from build123d import *

# Parameters (mm, degrees)
SKETCH1_W                      = 765
SKETCH1_H                      = 550
BASE_FLANGE1_DEPTH             = 1.8
EDGE_FLANGE1_STRIP_W           = 8.6732
EDGE_FLANGE1_STRIP_H           = 1.8
EDGE_FLANGE1_STRIP_CUT_DEPTH   = 550
EDGE_FLANGE1_STRIP_2_W         = 8.6732
EDGE_FLANGE1_STRIP_2_H         = 1.8
EDGE_FLANGE1_STRIP_CUT_2_DEPTH = 550
EDGE_FLANGE1_DEPTH             = 550
EDGE_FLANGE1_BEND_DEPTH        = 550
EDGE_FLANGE2_STRIP_W           = 8.6732
EDGE_FLANGE2_STRIP_H           = 1.8
EDGE_FLANGE2_STRIP_CUT_DEPTH   = 550
EDGE_FLANGE2_STRIP_2_W         = 8.6732
EDGE_FLANGE2_STRIP_2_H         = 1.8
EDGE_FLANGE2_STRIP_CUT_2_DEPTH = 550
EDGE_FLANGE2_DEPTH             = 550
EDGE_FLANGE2_BEND_DEPTH        = 550
SKETCH18_R                     = 3.5
CUT_EXTRUDE1_DEPTH             = 10


# Sheet-metal steps are written as plain solids
with BuildPart() as part:
    # Sketch1 → Base-Flange1 (new body)
    with BuildSketch(Plane(origin=(0, 0, 0), x_dir=(0, 0, -1), z_dir=(1, 0, 0))):
        Rectangle(SKETCH1_W, SKETCH1_H)
    extrude(amount=-BASE_FLANGE1_DEPTH)

    # Edge-Flange1 strip (across the edge) → Edge-Flange1 strip cut (cut)
    with BuildSketch(Plane(origin=(0, 275, 382.5), x_dir=(0, 0, -1), z_dir=(0, -1, 0))):
        with Locations((-1.8, -0.9)):
            Rectangle(EDGE_FLANGE1_STRIP_W, EDGE_FLANGE1_STRIP_H)
    extrude(amount=EDGE_FLANGE1_STRIP_CUT_DEPTH, mode=Mode.SUBTRACT)

    # Edge-Flange1 strip 2 (across the edge) → Edge-Flange1 strip cut 2 (cut)
    with BuildSketch(Plane(origin=(0, -275, -382.5), x_dir=(0, 0, 1), z_dir=(0, 1, 0))):
        with Locations((-1.8, -0.9)):
            Rectangle(EDGE_FLANGE1_STRIP_2_W, EDGE_FLANGE1_STRIP_2_H)
    extrude(amount=EDGE_FLANGE1_STRIP_CUT_2_DEPTH, mode=Mode.SUBTRACT)

    # Edge-Flange1 section (across the edge) → Edge-Flange1 (add)
    with BuildSketch(Plane(origin=(0, 275, 382.5), x_dir=(0, 0, -1), z_dir=(0, -1, 0))):
        with BuildLine():
            Line((0, 0.7366), (0, 48.2))
            Line((0, 48.2), (1.8, 48.2))
            Line((1.8, 48.2), (1.8, 0.7366))
            ThreePointArc((1.8, 0.7366), (2.015745145, 0.215745145), (2.5366, 0))
            Line((2.5366, 0), (2.5366, -1.8))
            ThreePointArc((2.5366, -1.8), (0.742952939, -1.057047061), (0, 0.7366))
        make_face()
    extrude(amount=EDGE_FLANGE1_DEPTH)

    # Edge-Flange1 section 2 (across the edge) → Edge-Flange1 bend (add)
    with BuildSketch(Plane(origin=(0, -275, -382.5), x_dir=(0, 0, 1), z_dir=(0, 1, 0))):
        with BuildLine():
            Line((0, 0.7366), (0, 48.2))
            Line((0, 48.2), (1.8, 48.2))
            Line((1.8, 48.2), (1.8, 0.7366))
            ThreePointArc((1.8, 0.7366), (2.015745145, 0.215745145), (2.5366, 0))
            Line((2.5366, 0), (2.5366, -1.8))
            ThreePointArc((2.5366, -1.8), (0.742952939, -1.057047061), (0, 0.7366))
        make_face()
    extrude(amount=EDGE_FLANGE1_BEND_DEPTH)

    # Edge-Flange2 strip (across the edge) → Edge-Flange2 strip cut (cut)
    with BuildSketch(Plane(origin=(48.2, 275, -382.5), x_dir=(-1, 0, 0), z_dir=(0, -1, 0))):
        with Locations((-3.6, -0.9)):
            Rectangle(EDGE_FLANGE2_STRIP_W, EDGE_FLANGE2_STRIP_H)
    extrude(amount=EDGE_FLANGE2_STRIP_CUT_DEPTH, mode=Mode.SUBTRACT)

    # Edge-Flange2 strip 2 (across the edge) → Edge-Flange2 strip cut 2 (cut)
    with BuildSketch(Plane(origin=(48.2, -275, 382.5), x_dir=(-1, 0, 0), z_dir=(0, 1, 0))):
        with Locations((-3.6, -0.9)):
            Rectangle(EDGE_FLANGE2_STRIP_2_W, EDGE_FLANGE2_STRIP_2_H)
    extrude(amount=EDGE_FLANGE2_STRIP_CUT_2_DEPTH, mode=Mode.SUBTRACT)

    # Edge-Flange2 section (across the edge) → Edge-Flange2 (add)
    with BuildSketch(Plane(origin=(48.2, 275, -382.5), x_dir=(-1, 0, 0), z_dir=(0, -1, 0))):
        with BuildLine():
            Line((-1.8, 0.7366), (-1.8, 28.2))
            Line((-1.8, 28.2), (0, 28.2))
            Line((0, 28.2), (0, 0.7366))
            ThreePointArc((0, 0.7366), (0.215745145, 0.215745145), (0.7366, 0))
            Line((0.7366, 0), (0.7366, -1.8))
            ThreePointArc((0.7366, -1.8), (-1.057047061, -1.057047061), (-1.8, 0.7366))
        make_face()
    extrude(amount=EDGE_FLANGE2_DEPTH)

    # Edge-Flange2 section 2 (across the edge) → Edge-Flange2 bend (add)
    with BuildSketch(Plane(origin=(48.2, -275, 382.5), x_dir=(-1, 0, 0), z_dir=(0, 1, 0))):
        with BuildLine():
            Line((-1.8, 0.7366), (-1.8, 28.2))
            Line((-1.8, 28.2), (0, 28.2))
            Line((0, 28.2), (0, 0.7366))
            ThreePointArc((0, 0.7366), (0.215745145, 0.215745145), (0.7366, 0))
            Line((0.7366, 0), (0.7366, -1.8))
            ThreePointArc((0.7366, -1.8), (-1.057047061, -1.057047061), (-1.8, 0.7366))
        make_face()
    extrude(amount=EDGE_FLANGE2_BEND_DEPTH)

    # Sketch18 → Cut-Extrude1 (cut)
    with BuildSketch(Plane.ZY.offset(-48.2)):
        with Locations((-396.9683, 221.5)):
            Circle(SKETCH18_R)
        with Locations((-396.9683, -221.5)):
            Circle(SKETCH18_R)
    cut_extrude1 = extrude(amount=-CUT_EXTRUDE1_DEPTH, mode=Mode.SUBTRACT)

    # Mirror1: Cut-Extrude1 across plane
    add(cut_extrude1.mirror(Plane.XY), mode=Mode.SUBTRACT)


solid = part.part
Could you check a few things on this model? Use its own coordinates, in mm. A direction names the side the tool comes from. Round coordinates to 2 decimals unless told otherwise and drop trailing zeros. Order: outer loops, then holes, each group sorted by start corner. A loop starts at its lowest first (then second) coordinate and runs counter-clockwise, first axis right, second up.
Q1. Please list where these lines run through material, in increasing order: probe 1 along Z at (x, y) = (22, -145); probe 2 along Z at (x, y) = (49, 221); probe 3 along Z at (x, y) = (48.7, -221.5).
Geometry says:
probe 1: z = -382.5 to -380.7, 380.7 to 382.5
probe 2: z = -410.7 to -400.43, -393.5 to -381.22, 381.22 to 393.5, 400.43 to 410.7
probe 3: z = -410.7 to -400.47, -393.47 to -381.02, 381.02 to 393.47, 400.47 to 410.7
Q2. Imagine slicing it at C-C, the plane z = 252.5. List the corners of the cut face in (x, y) for me.
Geometry says:
outline: (-1.8, -275) - (0, -275) - (0, 275) - (-1.8, 275) - close
Q3. I'm going to push flat-ended pins straight in: P1, Ø22, axis at y = -123, z = 402.5, coming from the -X side; P2, Ø2, axis at x = 39.5, y = -89, coming from the +Z side; P3, Ø5, axis at x = 44.5, y = 181, coming from the -Z side. Where does each tip first touch, or does it pass through?
Geometry says:
P1: stops at x = 48.2
P2: stops at z = 382.5
P3: stops at z = -382.5
Q4. Which directions (+Z, -Z, +X, -X, +Y, -Y) give clear straight access to the entire face, cutting with the end or side of a thin tool? Please do faces 4 (the face through (0, 4, 5)), 5 (the face through (48.2, 4, -397)), 6 (the face through (48.2, -4, 397)).
Geometry says:
face 4: +X, +Y, -Y
face 5: -Z, -X, +Y, -Y
face 6: +Z, -X, +Y, -Y
Q5. Imagine slicing it at B-B, the plane x = 29. List the corners of the cut face in (y, z) for me.
Geometry says:
outline: (-275, -382.5) - (275, -382.5) - (275, -380.7) - (-275, -380.7) - close; (-275, 380.7) - (275, 380.7) - (275, 382.5) - (-275, 382.5) - close
Q6. Thinking about a two-plate mould opening in Z: for faces 1 (the face through (24, 4, 382.5)), 2 (the face through (50, -4, 397)), 3 (the face through (24, -4, -380.7)), which applies, released by +Z, released by -Z, zero draft, split by the parting line, or undercut?
Geometry says:
face 1: released by +Z
face 2: zero draft
face 3: undercut
Q7. Imagine slicing it at A-A, the plane y = -51.5. List the corners of the cut face in (x, z) for me.
Geometry says:
outline: (-1.8, -379.96) arc R2.54 ccw to (0.74, -382.5) - (47.46, -382.5) arc R0.74 cw to (48.2, -383.24) - (48.2, -410.7) - (50, -410.7) - (50, -383.24) arc R2.54 ccw to (47.46, -380.7) - (0.74, -380.7) arc R0.74 cw to (0, -379.96) - (0, 379.96) arc R0.74 cw to (0.74, 380.7) - (47.46, 380.7) arc R2.54 ccw to (50, 383.24) - (50, 410.7) - (48.2, 410.7) - (48.2, 383.24) arc R0.74 cw to (47.46, 382.5) - (0.74, 382.5) arc R2.54 ccw to (-1.8, 379.96) - close
